Verification items for the finished model (mm, model axes). A direction names the side the tool comes from. Coordinates: 2 decimals unless noted, no trailing zeros. Write each loop counter-clockwise with the first axis right and the second up, starting at its lowest first coordinate (ties: lowest second). Pieces come first, ordered by that corner, then holes. Notation, with made-up numbers: (43, -20.75) -> (98, -20.75) arc R8 ccw to (98, -5.75) -> close; hole circle Ø7 at (-32.5, -32). An arc over 180 degrees is marked (long way). Answer in a Markdown table with one row per item.
```python
from build123d import *

# Parameters (mm, degrees)
SKETCH_1_W               = 1000
SKETCH_1_H               = 20
SKETCH_1_R               = 5
EXTRUDE_1_DEPTH          = 20
CUT_EXTRUDE_1_DEPTH      = 501.799361022
CUT_EXTRUDE_1_DEPTH_BACK = 20


with BuildPart() as part:
    # Эскиз1 → Бобышка-Вытянуть1 (new body)
    with BuildSketch(Plane.XY):
        Rectangle(SKETCH_1_W, SKETCH_1_H)
        with Locations((-490, 0)):
            Circle(SKETCH_1_R, mode=Mode.SUBTRACT)
        with Locations(Location((490, 0, 0), (0, 0, 180))):
            Circle(SKETCH_1_R, mode=Mode.SUBTRACT)
    extrude(amount=EXTRUDE_1_DEPTH)

    # Эскиз2 → Вырез-Вытянуть1 (cut, two sides: drawn at the far end of the back side and taken through both)
    with BuildSketch(Plane(origin=(0, 10, 0), x_dir=(1, 0, 0), z_dir=(0, 1, 0)).offset(-CUT_EXTRUDE_1_DEPTH_BACK)):
        Polygon((2510.224987345, -5), (500, -5), (470, -5), (470, -15), (500, -15), (2510.224987345, -15), (6530.674962036, -15), (6530.674962036, -5), align=None)
    extrude(amount=CUT_EXTRUDE_1_DEPTH + CUT_EXTRUDE_1_DEPTH_BACK, mode=Mode.SUBTRACT)


solid = part.part
```
1. Tool access check on faces 4 (the flat face through (-7, -10, 10)), 5 (the flat face through (485, -2, 5)). Record the directions out of +Z, -Z, +X, -X, +Y, -Y that give a thin tool (end or side, any length) a straight path to the whole face; none if there is none.
Geometry says:
| item | result |
|---|---|
| face 4 | +Z, -Z, +X, -X, -Y |
| face 5 | +X, +Y, -Y |
2. Thickness scan on line 1 (Y direction, x = 490, z = 3.25); line 2 (X direction, y = 9, z = 7.5); line 3 (X direction, y = 2, z = 9.5). Record the ranges inside material, lowest first. Write a range as from..to.
Geometry says:
| item | result |
|---|---|
| line 1 | -10..-5, 5..10 |
| line 2 | -500..470 |
| line 3 | -500..-494.58, -485.42..470 |
3. Section check A-A, the plane y = 0. Record the boundary of the cut face in (x, z), plus the area to 3 significant figures.
Geometry says:
| item | result |
|---|---|
| outline | (-500, 0) -> (-495, 0) -> (-495, 20) -> (-500, 20) -> close; (-485, 0) -> (485, 0) -> (485, 5) -> (470, 5) -> (470, 15) -> (485, 15) -> (485, 20) -> (-485, 20) -> close; (495, 0) -> (500, 0) -> (500, 5) -> (495, 5) -> close; (495, 15) -> (500, 15) -> (500, 20) -> (495, 20) -> close |
| area | 19,400 mm^2 |
4. Mould release check, pull along Z, two halves, no side actions. Record for faces 1 (the flat face through (-7, 0, 0)), 2 (the flat face through (484.8, -0.1, 15)), 3 (the flat face through (-7, 10, 10)): released by +Z, released by -Z, zero draft, split by the parting line, or undercut.
Geometry says:
| item | result |
|---|---|
| face 1 | released by -Z |
| face 2 | undercut |
| face 3 | zero draft |
5. Depth check by flat-ended pin: P1, Ø5, axis at y = 0, z = 10, coming from the +X side. Enter the tip coordinate at first touch or a pass-through.
Geometry says:
| item | result |
|---|---|
| P1 | x = 470 |
